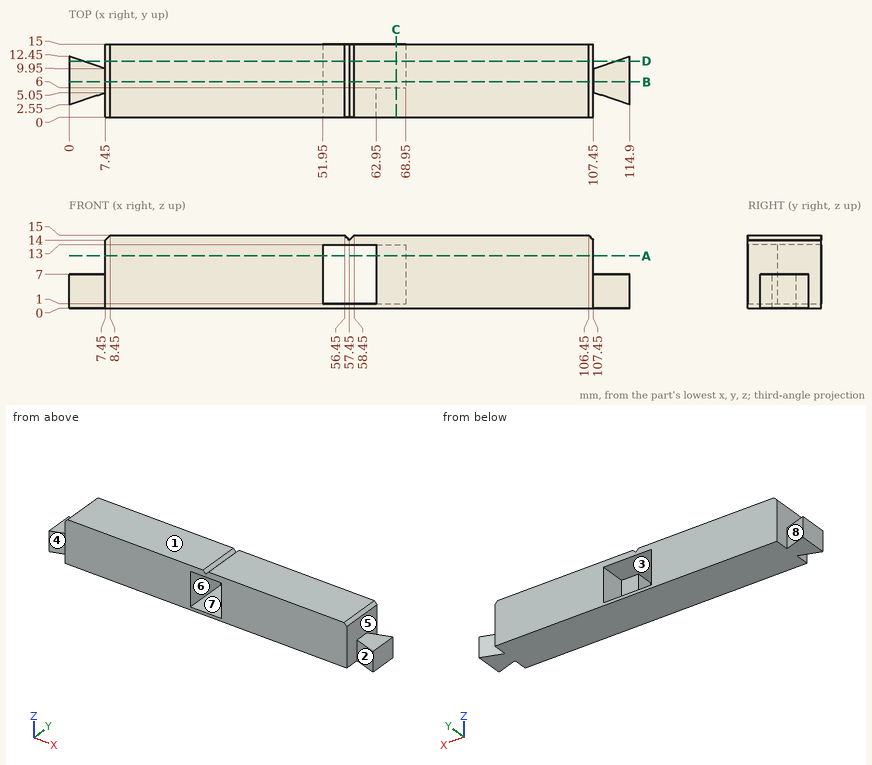
For this review, use the dimensioned drawing (mm, ordinates from the lowest corner) and the shaded views. A direction names the side the tool comes from. Coordinates: 2 decimals unless noted, no trailing zeros. Write each loop counter-clockwise with the first axis right and the second up, starting at its lowest first coordinate (ties: lowest second). Pieces come first, ordered by that corner, then holes. Notation, with made-up numbers: (0.25, 65.25) - (30.25, 65.25) arc R19 ccw to (30.25, 96.25) - close; hole circle Ø3 at (85.25, 17). An arc over 180 degrees is marked (long way). Answer in a Markdown table with one row per item. Add a question column.
Q1. Draft analysis for pull direction Z (two halves, no side actions). For the marked faces 1, 2 and 3, state which applies: +Z half, -Z half, draft (parallel to the pull), parting line (faces both ways), or undercut.
Q2. To check wall thickness, follow line 1 along X through (y, z) = (7.75, 12.25); line 2 along X through (y, z) = (3.25, 10); line 3 along Z through (x, y) = (55.5, 1.5). State the ranges of each line that lie inside material, in increasing order. Write a range as from..to.
Q3. Consider section A-A on z = 10.75. Give the boundary of the cut face in (x, y).
Q4. Consider section B-B on y = 7.25. Give the boundary of the cut face in (x, z).
Q5. Consider section C-C on x = 67. Give the boundary of the cut face in (y, z).
Q6. Consider section D-D on y = 11.5. Give the boundary of the cut face in (x, z).
Q7. For the marked faces 4, 5, 6, 7 and 8, list the 3-axis set-ups (+Z, -Z, +X, -X, +Y, -Y) from which the entire face can be reached by the end or side of a thin tool; tool diameter is ignored.
Q8. Clearance check with flat-ended pins moving along their axes: pin 1 (7 mm diameter, centred on y = 8, z = 5.5, fed in from -X); pin 2 (6 mm diameter, centred on x = 3, y = 5, fed in from +Z); pin 3 (1.8 mm diameter, centred on x = 66, z = 6.5, fed in from +Y); pin 4 (5 mm diameter, centred on y = 6, z = 13, fed in from -X). State where each tip first meets the part, or that it passes through.
Answers below:
| question | item | result |
|---|---|---|
| 1 | face 1 | +Z half |
| 1 | face 2 | draft |
| 1 | face 3 | undercut |
| 2 | line 1 | 7.45..51.95, 68.95..107.45 |
| 2 | line 2 | 7.45..51.95, 62.95..107.45 |
| 2 | line 3 | 0..1, 13..15 |
| 3 | outline | (7.45, 0) - (51.95, 0) - (51.95, 15) - (7.45, 15) - close; (62.95, 0) - (107.45, 0) - (107.45, 15) - (68.95, 15) - (68.95, 6) - (62.95, 6) - close |
| 4 | outline | (0, 0) - (114.9, 0) - (114.9, 7) - (107.45, 7) - (107.45, 14) - (106.45, 15) - (58.45, 15) - (57.45, 14) - (56.45, 15) - (8.45, 15) - (7.45, 14) - (7.45, 7) - (0, 7) - close; hole (51.95, 1) - (68.95, 1) - (68.95, 13) - (51.95, 13) - close |
| 5 | outline | (0, 0) - (15, 0) - (15, 1) - (6, 1) - (6, 13) - (15, 13) - (15, 15) - (0, 15) - close |
| 6 | outline | (0, 0) - (2.83, 0) - (2.83, 7) - (0, 7) - close; (7.45, 0) - (107.45, 0) - (107.45, 14) - (106.45, 15) - (58.45, 15) - (57.45, 14) - (56.45, 15) - (8.45, 15) - (7.45, 14) - close; (112.07, 0) - (114.9, 0) - (114.9, 7) - (112.07, 7) - close; hole (51.95, 1) - (68.95, 1) - (68.95, 13) - (51.95, 13) - close |
| 7 | face 4 | +Z, -Z, -Y |
| 7 | face 5 | +Z |
| 7 | face 6 | +Y, -Y |
| 7 | face 7 | +Y |
| 7 | face 8 | +Z, -Z, +Y |
| 8 | pin 1 | x = 0 |
| 8 | pin 2 | z = 7 |
| 8 | pin 3 | y = 6 |
| 8 | pin 4 | x = 7.45 |
